Source: CAD feature listing. Evaluate the final solid. Frame: model axes, mm. Face numbers are marked on the shaded views. A direction names the side the tool comes from. Round coordinates to 2 decimals unless told otherwise and drop trailing zeros. Order: outer loops, then holes, each group sorted by start corner. A loop starts at its lowest first (then second) coordinate and runs counter-clockwise, first axis right, second up. Notation, with made-up numbers: M 53.5,19.5 L 98.5,19.5 A15 ccw 98.5,26.5 Z; hole C -11.75,53 d5. An arc over 180 degrees is marked long. Use one line per item in the form item = value. Start each with the question number.
Q1. Section D-D (z = 6.5). Return the cut outline in (x, y), plus the area to 3 significant figures.
Q2. Section C-C (x = 45). Return the cut outline in (y, z), plus the area to 3 significant figures.
Q3. Pull-direction query (X, two-part tool) for the marked faces 4, 5, 6 and 7; classes: pulls with the +X half, pulls with the -X half, needs draft (parallel to the pull), parting line crosses it, or undercut.
Q4. Contact query for flat-ended pins moving along their axis: pin 1 (2.5 mm diameter, centred on x = 31, y = 25, fed in from -Z); pin 2 (4 mm diameter, centred on x = 27, y = 25.5, fed in from +Z); pin 3 (4 mm diameter, centred on x = 3.5, z = 5, fed in from +Y); pin 4 (3 mm diameter, centred on x = 27.5, z = 2, fed in from -Y). Output: stop coordinate, or through.
Q5. Section A-A (y = 5.75). Return the cut outline in (x, z).
Q6. Reachability of the marked faces 1, 2 and 3 from +Z, -Z, +X, -X, +Y, -Y: full face, straight path, thin tool, end or side. Return the list, or none.
Q7. Section B-B (z = 4). Give the number of separate pieces and of enclosed holes in the cut face, plus the area to 3 significant figures.
Q8. Material intervals for probe 1 along X at (y, z) = (1.35, 4); probe 2 along X at (y, z) = (10, 4.75); probe 3 along Y at (x, z) = (19, 3.45), sorted ascending.
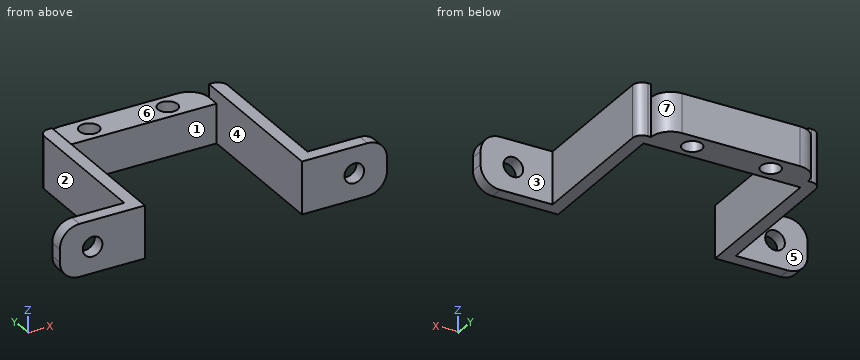
from build123d import *

# Parameters (mm, degrees)
EXTRUIR_L_MINA1_DEPTH   = 8
CROQUIS2_W              = 24
CROQUIS2_H              = 2
CORTAR_EXTRUIR1_DEPTH   = 2
CROQUIS3_W              = 24
CROQUIS3_H              = 6
SALIENTE_EXTRUIR1_DEPTH = 3
CROQUIS4_R              = 1.5
CORTAR_EXTRUIR2_DEPTH   = 58.621610529
CROQUIS5_R              = 1.5
CORTAR_EXTRUIR3_DEPTH   = 58.621610529
REDONDEO1_R             = 3
REDONDEO2_R             = 1.5


with BuildPart() as part:
    # Croquis1 → Extruir-Lámina1 (new body)
    with BuildSketch(Plane.XY):
        Polygon((0, 0), (13, 0), (13, 22.5), (37, 22.5), (37, 0), (50, 0), (50, 2), (39, 2), (39, 24.5), (11, 24.5), (11, 2), (0, 2), align=None)
    extrude(amount=EXTRUIR_L_MINA1_DEPTH)

    # Croquis2 → Cortar-Extruir1 (cut)
    with BuildSketch(Plane.XY.offset(8)):
        with Locations((25, 23.5)):
            Rectangle(CROQUIS2_W, CROQUIS2_H)
    extrude(amount=-CORTAR_EXTRUIR1_DEPTH, mode=Mode.SUBTRACT)

    # Croquis3 → Saliente-Extruir1 (add)
    with BuildSketch(Plane(origin=(0, 24.5, 0), x_dir=(1, 0, 0), z_dir=(0, 1, 0))):
        with Locations((25, -3)):
            Rectangle(CROQUIS3_W, CROQUIS3_H)
    extrude(amount=SALIENTE_EXTRUIR1_DEPTH)

    # Croquis4 → Cortar-Extruir2 (cut, through all)
    with BuildSketch(Plane(origin=(0, 0, 0), x_dir=(-1, 0, 0), z_dir=(0, 0, -1))):
        with Locations((-19, 25)):
            Circle(CROQUIS4_R)
        with Locations((-31, 25)):
            Circle(CROQUIS4_R)
    extrude(amount=-CORTAR_EXTRUIR2_DEPTH, mode=Mode.SUBTRACT)

    # Croquis5 → Cortar-Extruir3 (cut, through all)
    with BuildSketch(Plane.XZ):
        with Locations(Location((45, 4, 0), (0, 0, 270))):
            Circle(CROQUIS5_R)
        with Locations(Location((5, 4, 0), (0, 0, 90))):
            Circle(CROQUIS5_R)
    extrude(amount=-CORTAR_EXTRUIR3_DEPTH, mode=Mode.SUBTRACT)

    # Redondeo1
    redondeo1_edges = [part.edges().sort_by_distance(p)[0] for p in [
        (13, 27.5, 3),
        (37, 27.5, 3),
        (50, 1, 8),
        (50, 1, 0),
        (0, 1, 0),
        (0, 1, 8),
    ]]
    fillet(redondeo1_edges, radius=REDONDEO1_R - 0.0001)  # a hair under: the kernel refuses the full size

    # Redondeo2
    redondeo2_edges = [part.edges().sort_by_distance(p)[0] for p in [
        (11, 24.5, 4),
        (39, 24.5, 4),
    ]]
    fillet(redondeo2_edges, radius=REDONDEO2_R)


solid = part.part
Results list:
q1.outline = M 0.4,0 L 13,0 L 13,24.5 L 12.5,24.5 A1.5 ccw 11,23 L 11,2 L 0.4,2 Z; M 37,0 L 49.6,0 L 49.6,2 L 39,2 L 39,23 A1.5 ccw 37.5,24.5 L 37,24.5 Z
q1.area = 139 mm2
q2.outline = M 0,0 L 2,0 L 2,2.5 L 0,2.5 Z; M 0,5.5 L 2,5.5 L 2,8 L 0,8 Z
q2.area = 10.0 mm2
q3.face_4 = undercut
q3.face_5 = needs draft
q3.face_6 = undercut
q3.face_7 = pulls with the +X half
q4.pin_1 = through
q4.pin_2 = 6
q4.pin_3 = 2
q4.pin_4 = 22.5
q5.outline = M 11,0 L 13,0 L 13,8 L 11,8 Z; M 37,0 L 39,0 L 39,8 L 37,8 Z
q6.face_1 = +Z, -Z, -Y
q6.face_2 = +Z, -Z, -X, +Y
q6.face_3 = +Z, -Z, +X, +Y
q7.separate_pieces = 3
q7.enclosed_holes = 2
q7.area = 231 mm2
q8.probe_1 = 0 to 3.5, 6.5 to 13, 37 to 43.5, 46.5 to 50
q8.probe_2 = 11 to 13, 37 to 39
q8.probe_3 = 22.5 to 23.5, 26.5 to 27.5
